Geometry: final body of the model. Coordinates: model frame, mm. Coordinates: 2 decimals unless noted, no trailing zeros. Loops run counter-clockwise (first coordinate to the right, second up) from the corner with the lowest first, then second, coordinate; pieces in that order, holes last. Notation, with made-up numbers: (-12.5, 75.5) - (-3.5, 75.5) arc R18 ccw to (-3.5, 107.5) - close; hole circle Ø4 at (30, 54). An arc over 180 degrees is marked (long way). Return JSON: item names as keys, results as strings.
from build123d import *

# Parameters (mm, degrees)
SKETCH1_R           = 2.05
SKETCH1_R_2         = 3.5
SKETCH1_R_3         = 6
SKETCH1_R_4         = 1.55
SKETCH1_W           = 4
SKETCH1_H           = 8
BOSS_EXTRUDE1_DEPTH = 6.3
FILLET1_R           = 5


with BuildPart() as part:
    # Sketch1 → Boss-Extrude1 (new body)
    with BuildSketch(Plane(origin=(0, 0, 0), x_dir=(1, 0, 0), z_dir=(0, 1, 0))):
        Polygon((15, 94), (15, 59), (0, 59), (0, 0), (69, 0), (69, 59), (54, 59), (54, 94), align=None)
        with Locations(Location((9.5, 51.5, 0), (0, 0, 270))):
            Circle(SKETCH1_R, mode=Mode.SUBTRACT)
        with Locations(Location((59.5, 51.5, 0), (0, 0, 270))):
            Circle(SKETCH1_R, mode=Mode.SUBTRACT)
        with Locations(Location((9.5, 9, 0), (0, 0, 270))):
            Circle(SKETCH1_R_2, mode=Mode.SUBTRACT)
        with Locations(Location((59.5, 9, 0), (0, 0, 270))):
            Circle(SKETCH1_R_2, mode=Mode.SUBTRACT)
        with Locations(Location((24.5, 78, 0), (0, 0, 270))):
            Circle(SKETCH1_R_3, mode=Mode.SUBTRACT)
        with Locations(Location((44.5, 78, 0), (0, 0, 270))):
            Circle(SKETCH1_R_3, mode=Mode.SUBTRACT)
        with Locations(Location((34.5, 62, 0), (0, 0, 270))):
            Circle(SKETCH1_R_3, mode=Mode.SUBTRACT)
        with Locations(Location((34.5, 73.5, 0), (0, 0, 270))):
            Circle(SKETCH1_R_4, mode=Mode.SUBTRACT)
        with Locations(Location((26, 86, 0), (0, 0, 270))):
            Circle(SKETCH1_R_4, mode=Mode.SUBTRACT)
        with Locations(Location((43, 86, 0), (0, 0, 270))):
            Circle(SKETCH1_R_4, mode=Mode.SUBTRACT)
        with Locations((6, 30)):
            Rectangle(SKETCH1_W, SKETCH1_H, mode=Mode.SUBTRACT)
        with Locations((63, 30)):
            Rectangle(SKETCH1_W, SKETCH1_H, mode=Mode.SUBTRACT)
    extrude(amount=BOSS_EXTRUDE1_DEPTH)

    # Fillet1
    fillet1_edges = [part.edges().sort_by_distance(p)[0] for p in [
        (0, 3.15, -59),
        (15, 3.15, -59),
        (15, 3.15, -94),
        (54, 3.15, -94),
        (54, 3.15, -59),
        (69, 3.15, -59),
        (69, 3.15, 0),
        (0, 3.15, 0),
    ]]
    fillet(fillet1_edges, radius=FILLET1_R)


solid = part.part
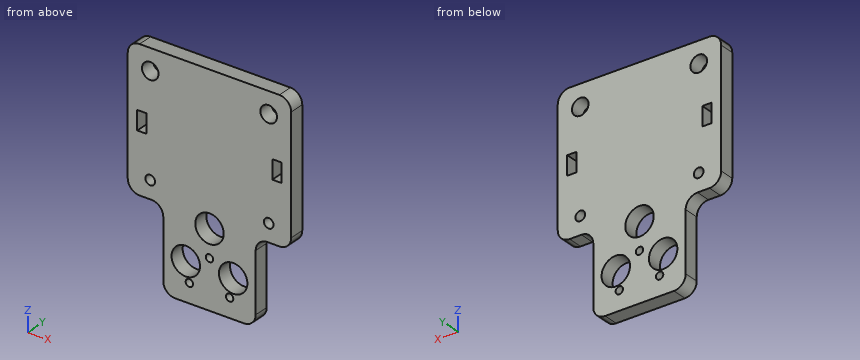
Item 1: Section query D-D, the plane z = -63. Return loops of the section in (x, y).
Worked out:
{"outline": "(14.9, 0) - (28.58, 0) - (28.58, 6.3) - (14.9, 6.3) - close; (40.42, 0) - (54.1, 0) - (54.1, 6.3) - (40.42, 6.3) - close"}
Item 2: Section query B-B, the plane z = -33. Return loops of the section in (x, y), and give its area (3 significant figures).
Worked out:
{"outline": "(0, 0) - (4, 0) - (4, 6.3) - (0, 6.3) - close; (8, 0) - (61, 0) - (61, 6.3) - (8, 6.3) - close; (65, 0) - (69, 0) - (69, 6.3) - (65, 6.3) - close", "area": "384 mm^2"}
Item 3: Ray query, probe 1 along X at (y, z) = (2.25, -86); probe 2 along X at (y, z) = (4.5, -51.5); probe 3 along Z at (x, y) = (58, 5.25). Return the intervals inside material, ascending. Write a range as from..to.
Worked out:
{"probe 1": "15..24.45, 27.55..41.45, 44.55..54", "probe 2": "0..7.45, 11.55..57.45, 61.55..69", "probe 3": "-59.1..-52.9, -50.1..-12.16, -5.84..0"}
Item 4: Section query A-A, the plane x = 34.5. Return loops of the section in (y, z).
Worked out:
{"outline": "(0, -94) - (6.3, -94) - (6.3, -75.05) - (0, -75.05) - close; (0, -71.95) - (6.3, -71.95) - (6.3, -68) - (0, -68) - close; (0, -56) - (6.3, -56) - (6.3, 0) - (0, 0) - close"}
Item 5: Section query C-C, the plane y = 2. Count the separate pieces of the cut face and the enclosed holes in it, and give its area (3 significant figures).
Worked out:
{"separate pieces": "1", "enclosed holes": "12", "area": "4,890 mm^2"}
Item 6: First-contact query: pin 1 Ø1.9 at (y, z) = (2.5, -80.5) entering from -X; pin 2 Ø3 at (x, y) = (6, 3.5) entering from -Z. Flat tips, straight axial feed; report the tip coordinate or a pass-through.
Worked out:
{"pin 1": "x = 15", "pin 2": "z = -59"}
